Design review of the part built by this model. Coordinates are the model's own, in mm. A direction names the side the tool comes from. Coordinates: 2 decimals unless noted, no trailing zeros. Loops run counter-clockwise (first coordinate to the right, second up) from the corner with the lowest first, then second, coordinate; pieces in that order, holes last. Notation, with made-up numbers: (-21, 48) - (18, 48) arc R37 cw to (18, 86) - close; hole circle Ø8 at (-34.75, 29.5). An arc over 180 degrees is marked (long way). Use one line per item in the form item = value. Start each with the question number.
(1) Add section B-B (y = 7.5). State the section outline as (x, z) points (3 decimals), plus the area to 3 significant figures.
(2) Add section A-A (x = 25.4). State the section outline as (y, z) points (3 decimals), plus the area to 3 significant figures.
(3) Add section D-D (z = 2.15). State the section outline as (x, y) points (3 decimals), plus the area to 3 significant figures.
(4) The part is to be moulded in two halves that separate along Y. For faces 3 (the face through (50.8, 20, 2)), 4 (the face through (38, 9.525, 2)), 5 (the face through (25, 0, 2)), say which applies: pulls with the +Y half, pulls with the -Y half, needs draft (parallel to the pull), parting line crosses it, or undercut.
(5) For L1, parallel to X at y = 9, z = 2.35; L2, parallel to Y at x = 9.5, z = 0.4 (3 decimals); L3, parallel to Y at x = 25.4, z = 1.8 (3 decimals), list the stretches that pass through material, from the lowest coordinate up.
(6) Add section C-C (y = 24). State the section outline as (x, z) points (3 decimals), plus the area to 3 significant figures.
(7) Tool access review of faces 1 (the face through (31.75, 8, 2)), 2 (the face through (2.29, 45.45, 1.57)): name each direction out of +Z, -Z, +X, -X, +Y, -Y from which nothing blocks a thin tool from reaching the whole face with its end or side.
```python
from build123d import *

# Parameters (mm, degrees)
SKETCH1_R           = 8.5
SKETCH1_W           = 12.7
SKETCH1_H           = 3.175
BOSS_EXTRUDE1_DEPTH = 3.175


with BuildPart() as part:
    # Sketch1 → Boss-Extrude1 (new body)
    with BuildSketch(Plane.XY):
        with BuildLine():
            Line((50.8, 0), (50.8, 40.005))
            ThreePointArc((50.8, 40.005), (48.568153673, 45.393153673), (43.18, 47.625))
            Line((43.18, 47.625), (7.62, 47.625))
            ThreePointArc((7.62, 47.625), (2.231846327, 45.393153673), (0, 40.005))
            Line((0, 40.005), (0, 0))
            Line((0, 0), (50.8, 0))
        make_face()
        with Locations((25.4, 28.575)):
            Circle(SKETCH1_R, mode=Mode.SUBTRACT)
        with Locations((12.7, 7.9375)):
            Rectangle(SKETCH1_W, SKETCH1_H, mode=Mode.SUBTRACT)
        with Locations((38.1, 7.9375)):
            Rectangle(SKETCH1_W, SKETCH1_H, mode=Mode.SUBTRACT)
    extrude(amount=BOSS_EXTRUDE1_DEPTH)


solid = part.part
```
Computed values:
q1.outline = (0, 0) - (6.35, 0) - (6.35, 3.175) - (0, 3.175) - close; (19.05, 0) - (31.75, 0) - (31.75, 3.175) - (19.05, 3.175) - close; (44.45, 0) - (50.8, 0) - (50.8, 3.175) - (44.45, 3.175) - close
q1.area = 80.6 mm^2
q2.outline = (0, 0) - (20.075, 0) - (20.075, 3.175) - (0, 3.175) - close; (37.075, 0) - (47.625, 0) - (47.625, 3.175) - (37.075, 3.175) - close
q2.area = 97.2 mm^2
q3.outline = (0, 0) - (50.8, 0) - (50.8, 40.005) arc R7.62 ccw to (43.18, 47.625) - (7.62, 47.625) arc R7.62 ccw to (0, 40.005) - close; hole (6.35, 6.35) - (19.05, 6.35) - (19.05, 9.525) - (6.35, 9.525) - close; hole circle Ø17 at (25.4, 28.575); hole (31.75, 6.35) - (44.45, 6.35) - (44.45, 9.525) - (31.75, 9.525) - close
q3.area = 2,090 mm^2
q4.face_3 = needs draft
q4.face_4 = undercut
q4.face_5 = pulls with the -Y half
q5.L1 = 0 to 6.35, 19.05 to 31.75, 44.45 to 50.8
q5.L2 = 0 to 6.35, 9.525 to 47.625
q5.L3 = 0 to 20.075, 37.075 to 47.625
q6.outline = (0, 0) - (18.236, 0) - (18.236, 3.175) - (0, 3.175) - close; (32.564, 0) - (50.8, 0) - (50.8, 3.175) - (32.564, 3.175) - close
q6.area = 116 mm^2
q7.face_1 = +Z, -Z
q7.face_2 = +Z, -Z, -X, +Y
